Can you work these out from the model? Positions are in its coordinate system, mm. A direction names the side the tool comes from. Coordinates: 2 decimals unless noted, no trailing zeros. Order: outer loops, then holes, each group sorted by start corner. A loop starts at its lowest first (then second) coordinate and runs counter-clockwise, first axis right, second up. Notation, with made-up numbers: (-13, 85.5) -> (-8, 85.5) arc R16 ccw to (-8, 106.5) -> close; hole circle Ø4 at (87, 68). An arc over 180 degrees is marked (long way). Answer in a Markdown table with one row per item. Add a question column.
1. Will these pins go through, and if not, where does the flat tip stop? pin 1 (1.5 mm diameter, centred on y = 51, z = 0, fed in from -X); pin 2 (3.5 mm diameter, centred on x = 2.5, y = 84, fed in from +Z); pin 3 (3 mm diameter, centred on x = -7, y = 29.5, fed in from -Z); pin 4 (12 mm diameter, centred on x = -4, z = 8.5, fed in from +Y) (3 decimals).
2. If I drill on line 1 along Y through (x, z) = (0, 12) (3 decimals); line 2 along Y through (x, z) = (-4, 2.75); line 3 along Z through (x, y) = (3.5, 50), over which ranges is the centre line in solid material (lowest first)? Write a range as [from, to].
3. On a 3-axis mill with a long thin cutter (end or side, diameter ignored), from which of +Z, -Z, +X, -X, +Y, -Y can I reach the whole of each face in a straight line? I mean faces 3 (the face through (-8.44, 75.31, 11.55)), 4 (the face through (8.379, 77.089, 1.086)), 5 (the face through (0, 77, 12.7)), 6 (the face through (0, 77, 0)), 7 (the face through (9.525, 77, 6)). Say none if no direction works.
4. Imagine slicing it at D-D on x = -8. State how many separate pieces and enclosed holes the cut face has, plus the area to 3 significant figures.
5. Imagine slicing it at C-C on y = 29.5. Write out the boundary of the cut face in (x, z) (3 decimals).
6. We'd pull the mould along Y, two halves only. Please class faces 1 (the face through (9, 156, -6.35)), 2 (the face through (-8.379, 75.311, 1.086)): pulls with the +Y half, pulls with the -Y half, needs draft (parallel to the pull), parting line crosses it, or undercut.
7. Imagine slicing it at B-B on z = 7.25. Write out the boundary of the cut face in (x, y) (3 decimals), plus the area to 3 significant figures.
8. Imagine slicing it at A-A on x = 0. Write out the boundary of the cut face in (y, z) (3 decimals), plus the area to 3 significant figures.
from build123d import *
from build123d.topology import SkipClean

# Parameters (mm, degrees)
BOSS_EXTRUDE1_DEPTH      = 12.7
BOSS_EXTRUDE2_DEPTH      = 6.35
BOSS_EXTRUDE2_DEPTH_BACK = 19.05
SKETCH3_R                = 15.875
FILLET1_R                = 3.81
SKETCH4_R                = 9.525
CUT_EXTRUDE1_DEPTH       = 52.578
CHAMFER1_SIZE            = 2.54


with BuildPart() as part:
    # Sketch2 → Boss-Extrude1 (new body)
    with BuildSketch(Plane.XY):
        with BuildLine():
            Line((-9.525, 12.7), (-9.525, 139.7))
            ThreePointArc((-9.525, 139.7), (0, 168.275), (9.525, 139.7))
            Line((9.525, 139.7), (9.525, 12.7))
            ThreePointArc((9.525, 12.7), (0, -15.875), (-9.525, 12.7))
        make_face()
    extrude(amount=BOSS_EXTRUDE1_DEPTH)

    # Sketch3 → Boss-Extrude2 (add, two sides: drawn at the far end of the back side and taken through both)
    with SkipClean():  # the faces are left unmerged after this step: merging them gives an invalid solid
        with BuildSketch(Plane(origin=(0, 0, 0), x_dir=(-1, 0, 0), z_dir=(0, 0, -1)).offset(-BOSS_EXTRUDE2_DEPTH_BACK)):
            with Locations((0, 152.4)):
                Circle(SKETCH3_R)
            Circle(SKETCH3_R)
        extrude(amount=BOSS_EXTRUDE2_DEPTH + BOSS_EXTRUDE2_DEPTH_BACK)
    add(part.part.scale(1), mode=Mode.REPLACE)  # the faces are merged on a copy

    # Fillet1
    # the kernel refuses this fillet: 3.81 mm, written as the material it takes off along each edge
    with BuildSketch(Plane(origin=(-9.525, 3.175, 12.7), x_dir=(1, 0, 0), z_dir=(0, 1, 0))) as fillet1_piece_1_section:
        with BuildLine():
            CenterArc((FILLET1_R, FILLET1_R), FILLET1_R, 180, 90)
            Line((0, FILLET1_R), (0, 0))
            Line((0, 0), (FILLET1_R, 0))
        make_face()
    fillet1_piece_1 = extrude(amount=146.05, mode=Mode.PRIVATE)
    fillet1_piece_1 = fillet1_piece_1 - Plane(origin=(0, 152.4, 11.833457617), x_dir=(-1, 0, 0), z_dir=(0, 0, -1)) * Cylinder(15.875, 308, mode=Mode.PRIVATE)
    fillet1_piece_1 = fillet1_piece_1 - Plane(origin=(0, 0, 11.833457617), x_dir=(-1, 0, 0), z_dir=(0, 0, -1)) * Cylinder(15.875, 308, mode=Mode.PRIVATE)
    add(fillet1_piece_1, mode=Mode.SUBTRACT)
    with BuildSketch(Plane(origin=(-9.525, 3.175, 0), x_dir=(1, 0, 0), z_dir=(0, 1, 0))) as fillet1_piece_2_section:
        with BuildLine():
            CenterArc((FILLET1_R, -FILLET1_R), FILLET1_R, 90, 90)
            Line((0, -FILLET1_R), (0, 0))
            Line((0, 0), (FILLET1_R, 0))
        make_face()
    fillet1_piece_2 = extrude(amount=146.05, mode=Mode.PRIVATE)
    fillet1_piece_2 = fillet1_piece_2 - Plane(origin=(0, 152.4, 0.866542383), x_dir=(-1, 0, 0), z_dir=(0, 0, 1)) * Cylinder(15.875, 308, mode=Mode.PRIVATE)
    fillet1_piece_2 = fillet1_piece_2 - Plane(origin=(0, 0, 0.866542383), x_dir=(-1, 0, 0), z_dir=(0, 0, 1)) * Cylinder(15.875, 308, mode=Mode.PRIVATE)
    add(fillet1_piece_2, mode=Mode.SUBTRACT)
    with BuildSketch(Plane(origin=(9.525, 149.225, 0), x_dir=(0, 0, 1), z_dir=(0, -1, 0))) as fillet1_piece_3_section:
        with BuildLine():
            CenterArc((FILLET1_R, FILLET1_R), FILLET1_R, 180, 90)
            Line((0, FILLET1_R), (0, 0))
            Line((0, 0), (FILLET1_R, 0))
        make_face()
    fillet1_piece_3 = extrude(amount=146.05, mode=Mode.PRIVATE)
    fillet1_piece_3 = fillet1_piece_3 - Plane(origin=(0, 152.4, 0.866542379), x_dir=(-0.5999999999999995, -0.8000000000000005, 0), z_dir=(0, 0, -1)) * Cylinder(15.875, 308, mode=Mode.PRIVATE)
    fillet1_piece_3 = fillet1_piece_3 - Plane(origin=(0, 0, 0.866542379), x_dir=(0.6000000000000001, 0.7999999999999999, 0), z_dir=(0, 0, -1)) * Cylinder(15.875, 308, mode=Mode.PRIVATE)
    add(fillet1_piece_3, mode=Mode.SUBTRACT)
    with BuildSketch(Plane(origin=(9.525, 149.225, 12.7), x_dir=(0, 0, -1), z_dir=(0, -1, 0))) as fillet1_piece_4_section:
        with BuildLine():
            CenterArc((FILLET1_R, -FILLET1_R), FILLET1_R, 90, 90)
            Line((0, -FILLET1_R), (0, 0))
            Line((0, 0), (FILLET1_R, 0))
        make_face()
    fillet1_piece_4 = extrude(amount=146.05, mode=Mode.PRIVATE)
    fillet1_piece_4 = fillet1_piece_4 - Plane(origin=(0, 152.4, 11.833457621), x_dir=(-0.5999999999999995, -0.8000000000000005, 0), z_dir=(0, 0, -1)) * Cylinder(15.875, 308, mode=Mode.PRIVATE)
    fillet1_piece_4 = fillet1_piece_4 - Plane(origin=(0, 0, 11.833457621), x_dir=(0.6000000000000001, 0.7999999999999999, 0), z_dir=(0, 0, -1)) * Cylinder(15.875, 308, mode=Mode.PRIVATE)
    add(fillet1_piece_4, mode=Mode.SUBTRACT)

    # Sketch4 → Cut-Extrude1 (cut)
    with BuildSketch(Plane(origin=(0, 0, -6.35), x_dir=(-1, 0, 0), z_dir=(0, 0, -1))):
        with Locations((0, 152.4)):
            Circle(SKETCH4_R)
        Circle(SKETCH4_R)
    extrude(amount=-CUT_EXTRUDE1_DEPTH, mode=Mode.SUBTRACT)

    # Chamfer1
    chamfer1_edges = [part.edges().sort_by_distance(p)[0] for p in [
        (15.875, 152.4, 19.05),
        (15.875, 152.4, -6.35),
        (15.875, 0, 19.05),
        (15.875, 0, -6.35),
    ]]
    chamfer(chamfer1_edges, length=CHAMFER1_SIZE)


solid = part.part
Answers follow:
| question | item | result |
|---|---|---|
| 1 | pin 1 | stops at x = -7.98 |
| 1 | pin 2 | stops at z = 12.7 |
| 1 | pin 3 | stops at z = 0 |
| 1 | pin 4 | stops at y = 168.275 |
| 2 | line 1 | y = [-15.875, -9.525], [9.525, 142.875], [161.925, 168.275] |
| 2 | line 2 | y = [-15.36, -8.64], [8.64, 143.76], [161.04, 167.76] |
| 2 | line 3 | z = [0, 12.7] |
| 3 | face 3 | +Z, -X |
| 3 | face 4 | -Z, +X |
| 3 | face 5 | +Z, +X, -X |
| 3 | face 6 | -Z, +X, -X |
| 3 | face 7 | +Z, -Z, +X |
| 4 | separate pieces | 3 |
| 4 | enclosed holes | 0 |
| 4 | area | 2,230 mm² |
| 5 | outline | (-9.525, 3.81) arc R3.81 ccw to (-5.715, 0) -> (5.715, 0) arc R3.81 ccw to (9.525, 3.81) -> (9.525, 8.89) arc R3.81 ccw to (5.715, 12.7) -> (-5.715, 12.7) arc R3.81 ccw to (-9.525, 8.89) -> close |
| 6 | face 1 | needs draft |
| 6 | face 2 | undercut |
| 7 | outline | (-9.525, 12.7) arc R15.875 ccw (long way) to (9.525, 12.7) -> (9.525, 139.7) arc R15.875 ccw (long way) to (-9.525, 139.7) -> close; hole circle Ø19.05 at (0, 0); hole circle Ø19.05 at (0, 152.4) |
| 7 | area | 3,350 mm² |
| 8 | outline | (-15.875, -3.81) -> (-13.335, -6.35) -> (-9.525, -6.35) -> (-9.525, 19.05) -> (-13.335, 19.05) -> (-15.875, 16.51) -> close; (9.525, -6.35) -> (13.335, -6.35) -> (15.875, -3.81) -> (15.875, 0) -> (136.525, 0) -> (136.525, -3.81) -> (139.065, -6.35) -> (142.875, -6.35) -> (142.875, 19.05) -> (139.065, 19.05) -> (136.525, 16.51) -> (136.525, 12.7) -> (15.875, 12.7) -> (15.875, 16.51) -> (13.335, 19.05) -> (9.525, 19.05) -> close; (161.925, -6.35) -> (165.735, -6.35) -> (168.275, -3.81) -> (168.275, 16.51) -> (165.735, 19.05) -> (161.925, 19.05) -> close |
| 8 | area | 2,150 mm² |
